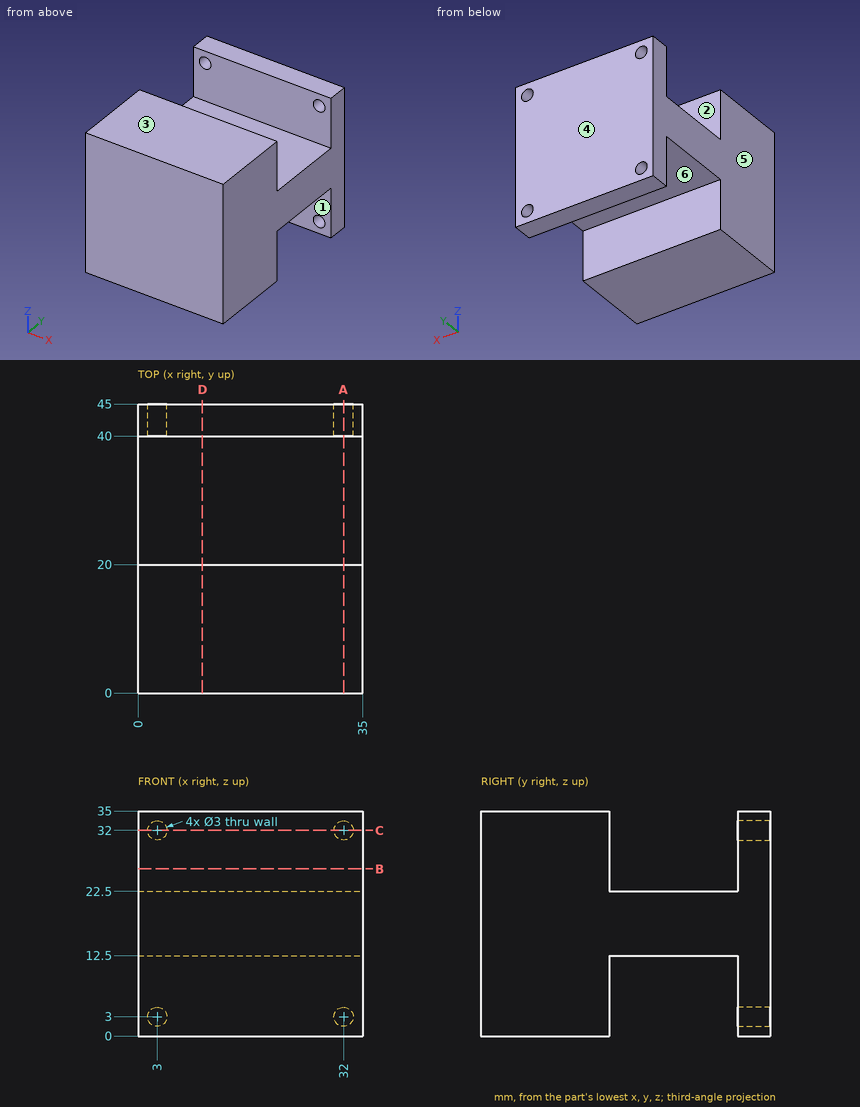
Study the drawing (mm; zero at the part's minimum x, y, z) and answer. A direction names the side the tool comes from. Coordinates: 2 decimals unless noted, no trailing zeros. Loops run counter-clockwise (first coordinate to the right, second up) from the corner with the lowest first, then second, coordinate; pieces in that order, holes last. Notation, with made-up numbers: M 87.5,16 L 96.5,16 A15 ccw 96.5,33 Z; hole C -11,78 d1. An arc over 180 degrees is marked long. Answer in a Markdown table with one row per item.
1) Find section A-A (x = 32). Determine the outline of the cut face in (y, z).
Answers below:
| item | result |
|---|---|
| outline | M 0,0 L 20,0 L 20,12.5 L 40,12.5 L 40,4.5 L 45,4.5 L 45,30.5 L 40,30.5 L 40,22.5 L 20,22.5 L 20,35 L 0,35 Z; M 40,0 L 45,0 L 45,1.5 L 40,1.5 Z; M 40,33.5 L 45,33.5 L 45,35 L 40,35 Z |
2) Find section B-B (z = 26). Determine the outline of the cut face in (x, y).
Answers below:
| item | result |
|---|---|
| outline | M 0,0 L 35,0 L 35,20 L 0,20 Z; M 0,40 L 35,40 L 35,45 L 0,45 Z |
3) Determine the mould class of the marked faces 4, 5 and 6 for opening direction Y: released by +Y, released by -Y, zero draft, split by the parting line, or undercut.
Answers below:
| item | result |
|---|---|
| face 4 | released by +Y |
| face 5 | zero draft |
| face 6 | undercut |
4) Find section D-D (x = 10). Determine the outline of the cut face in (y, z), then the cut area to 4 significant figures.
Answers below:
| item | result |
|---|---|
| outline | M 0,0 L 20,0 L 20,12.5 L 40,12.5 L 40,0 L 45,0 L 45,35 L 40,35 L 40,22.5 L 20,22.5 L 20,35 L 0,35 Z |
| area | 1,075 mm^2 |
5) Which of the six approach directions +Z, -Z, +X, -X, +Y, -Y give full straight-line access (tool end or side, diameter ignored) to the marked faces 1, 2 and 3?
Answers below:
| item | result |
|---|---|
| face 1 | -Z, +X, -X |
| face 2 | +Z, +X, -X |
| face 3 | +Z, +X, -X, +Y, -Y |
6) Find section C-C (z = 32). Determine the outline of the cut face in (x, y), then the cut area to 3 significant figures.
Answers below:
| item | result |
|---|---|
| outline | M 0,0 L 35,0 L 35,20 L 0,20 Z; M 0,40 L 1.5,40 L 1.5,45 L 0,45 Z; M 4.5,40 L 30.5,40 L 30.5,45 L 4.5,45 Z; M 33.5,40 L 35,40 L 35,45 L 33.5,45 Z |
| area | 845 mm^2 |
7) Given pin 1 (6 mm diameter, centred on x = 15, y = 29.5, fed in from -Z); pin 2 (1.8 mm diameter, centred on x = 32, z = 3, fed in from +Y); pin 3 (2 mm diameter, centred on x = 20, y = 31.5, fed in from +Z), each flat-ended and moving along its own axis, determine where each tip first touches the part or whether it passes through.
Answers below:
| item | result |
|---|---|
| pin 1 | z = 12.5 |
| pin 2 | y = 20 |
| pin 3 | z = 22.5 |
8) Find the intervals of material crossed by probe 1 along X at (y, z) = (43.45, 32); probe 2 along Y at (x, z) = (10, 5.5); probe 3 along Z at (x, y) = (21, 29), in increasing order.
Answers below:
| item | result |
|---|---|
| probe 1 | 0 to 1.5, 4.5 to 30.5, 33.5 to 35 |
| probe 2 | 0 to 20, 40 to 45 |
| probe 3 | 12.5 to 22.5 |
